```python
from build123d import *

# Parameters (mm, degrees)
SKETCH_1_R          = 3.175
EXTRUDE_1_DEPTH     = 57.15
CUT_EXTRUDE_1_DEPTH = 10.795
SKETCH_3_R          = 0.889
CUT_EXTRUDE_2_DEPTH = 10.795
SKETCH_4_W          = 3.926157487
SKETCH_4_H          = 0.79375
CUT_EXTRUDE_3_DEPTH = 8.573
SKETCH_5_R          = 3.774888962
CUT_EXTRUDE_4_DEPTH = 11.4


with BuildPart() as part:
    # 草图1 → 凸台-拉伸1 (new body)
    with BuildSketch(Plane(origin=(0, 0, 0), x_dir=(1, 0, 0), z_dir=(0, 1, 0))):
        Circle(SKETCH_1_R)
    extrude(amount=EXTRUDE_1_DEPTH)

    # 草图2 → 切除-拉伸1 (cut)
    with BuildSketch(Plane(origin=(0, 57.15, 0), x_dir=(1, 0, 0), z_dir=(0, 1, 0))):
        Polygon((-0.794, 3.175), (0.794, 3.175), (0.794, -3.175), (-3.175, -3.175), (-3.175, 3.175), align=None)
    extrude(amount=-CUT_EXTRUDE_1_DEPTH, mode=Mode.SUBTRACT)

    # 草图3 → 切除-拉伸2 (cut)
    with BuildSketch(Plane.ZY.offset(-0.794)):
        with Locations((0, 53.855)):
            Circle(SKETCH_3_R)
        with Locations((0, 48.855)):
            Circle(SKETCH_3_R)
    extrude(amount=-CUT_EXTRUDE_2_DEPTH, mode=Mode.SUBTRACT)

    # 草图4 → 切除-拉伸3 (cut)
    with BuildSketch(Plane.XZ):
        with Locations((-0.018009896, -2.778125)):
            Rectangle(SKETCH_4_W, SKETCH_4_H)
    extrude(amount=-CUT_EXTRUDE_3_DEPTH, mode=Mode.SUBTRACT)

    # 草图5 → 切除-拉伸4 (cut)
    with BuildSketch(Plane.XZ):
        Circle(SKETCH_5_R)
    extrude(amount=-CUT_EXTRUDE_4_DEPTH, mode=Mode.SUBTRACT)


solid = part.part
```
Can you work these out from the model? Positions are in its coordinate system, mm. A direction names the side the tool comes from. Coordinates: 2 decimals unless noted, no trailing zeros. Write each loop counter-clockwise with the first axis right and the second up, starting at its lowest first coordinate (ties: lowest second). Pieces come first, ordered by that corner, then holes. Notation, with made-up numbers: M 87.5,87.25 L 107.5,87.25 A34 ccw 107.5,120.25 Z; hole C 58.25,65 d11. An arc over 180 degrees is marked long. Write item = value, one per line. Start each with the question number.
Q1. If we section it at D-D, the plane x = 0: Write out the boundary of the cut face in (y, z) (3 decimals), then the cut area to 3 significant figures.
Q2. On a 3-axis mill with a long thin cutter (end or side, diameter ignored), from which of +Z, -Z, +X, -X, +Y, -Y can I reach the whole of each face in a straight line? I mean faces 1 (the face through (0.794, 52, 0)), 2 (the face through (3.03, 33.95, -0.95)). Say none if no direction works.
Q3. If we section it at C-C, the plane y = 15: Write out the boundary of the cut face in (x, z) (3 decimals), then the cut area to 3 significant figures.
Q4. If I drill on L1, parallel to Y at x = 2.5, z = 0; L2, parallel to Y at x = 0.75, z = 1.5 (3 decimals); L3, parallel to Y at x = 2.25, z = -0.75, over which ranges is the centre line in solid material (lowest first)? Write a range as [from, to].
Q5. If we section it at A-A, the plane z = 0: Write out the boundary of the cut face in (x, y) (3 decimals), then the cut area to 3 significant figures.
Q6. Thinking about a two-plate mould opening in Y: for faces 3 (the face through (1.968, 47.987, -0.193)), 4 (the face through (0, 11.4, 0)), 5 (the face through (2, 57.15, 0)), which applies, released by +Y, released by -Y, zero draft, split by the parting line, or undercut?
Q7. I'm going to push flat-ended pins straight in: pin 1 (3 mm diameter, centred on y = 45.5, z = 1.5, fed in from -X) (3 decimals); pin 2 (1.4 mm diameter, centred on y = 53.855, z = 0, fed in from +X). Where does each tip first touch, or does it pass through?
Q8. If we section it at B-B, the plane x = 2.5: Write out the boundary of the cut face in (y, z) (3 decimals).
Check sheet entries:
q1.outline = M 11.4,-3.175 L 46.355,-3.175 L 46.355,3.175 L 11.4,3.175 Z
q1.area = 222 mm²
q2.face_1 = +Z, -Z, -X, +Y
q2.face_2 = +Y, -Y
q3.outline = C 0,0 d6.35
q3.area = 31.7 mm²
q4.L1 = [11.4, 47.97], [49.74, 52.97], [54.74, 57.15]
q4.L2 = [11.4, 46.355]
q4.L3 = [11.4, 48.38], [49.33, 53.38], [54.33, 57.15]
q5.outline = M -3.175,11.4 L 3.175,11.4 L 3.175,47.966 L 0.794,47.966 L 0.794,46.355 L -3.175,46.355 Z; M 0.794,49.744 L 3.175,49.744 L 3.175,52.966 L 0.794,52.966 Z; M 0.794,54.744 L 3.175,54.744 L 3.175,57.15 L 0.794,57.15 Z
q5.area = 239 mm²
q6.face_3 = undercut
q6.face_4 = released by -Y
q6.face_5 = released by +Y
q7.pin_1 = -3.175
q7.pin_2 = through
q8.outline = M 11.4,-1.957 L 57.15,-1.957 L 57.15,1.957 L 11.4,1.957 Z; hole C 48.855,0 d1.778; hole C 53.855,0 d1.778
